Geometry: final body of the model. Coordinates: model frame, mm. Face numbers are marked on the shaded views. A direction names the side the tool comes from. Round coordinates to 2 decimals unless told otherwise and drop trailing zeros. Loops run counter-clockwise (first coordinate to the right, second up) from the corner with the lowest first, then second, coordinate; pieces in that order, holes last. Notation, with made-up numbers: (-31, 84.5) -> (1, 84.5) arc R11 ccw to (1, 100.5) -> close; hole circle Ø6 at (70.25, 56). An arc over 180 degrees is marked (long way). Answer in a Markdown table with one row per item.
```python
from build123d import *

# Parameters (mm, degrees)
SKETCH2_R           = 1.5
BOSS_EXTRUDE1_DEPTH = 10.5
SKETCH3_R           = 8
CUT_EXTRUDE1_DEPTH  = 4.5
SKETCH5_R           = 1.5
CUT_EXTRUDE3_DEPTH  = 22.113593143
CUT_EXTRUDE2_START  = -3
SKETCH4_R           = 8
CUT_EXTRUDE2_DEPTH  = 3


with BuildPart() as part:
    # Sketch2 → Boss-Extrude1 (new body)
    with BuildSketch(Plane.XY):
        with BuildLine():
            Line((7.937253933, 9), (14, 9))
            Line((14, 9), (14, -9))
            Line((14, -9), (7.937253933, -9))
            ThreePointArc((7.937253933, -9), (6.576406328, -10.037473776), (5.081826677, -10.870834265))
            Line((5.081826677, -10.870834265), (5.081826677, -16))
            Line((5.081826677, -16), (0, -16))
            Line((0, -16), (0, -9))
            Line((0, -9), (0, -6))
            ThreePointArc((0, -6), (6, 0), (0, 6))
            Line((0, 6), (0, 9))
            Line((0, 9), (0, 16))
            Line((0, 16), (5.081826677, 16))
            Line((5.081826677, 16), (5.081826677, 10.870834265))
            ThreePointArc((5.081826677, 10.870834265), (6.576406328, 10.037473776), (7.937253933, 9))
        make_face()
        with Locations(Location((10, 5, 0), (0, 0, 180))):
            Circle(SKETCH2_R, mode=Mode.SUBTRACT)
        with Locations(Location((10, -5, 0), (0, 0, 180))):
            Circle(SKETCH2_R, mode=Mode.SUBTRACT)
    extrude(amount=BOSS_EXTRUDE1_DEPTH)

    # Sketch3 → Cut-Extrude1 (cut)
    with BuildSketch(Plane.XY.offset(10.5)):
        Circle(SKETCH3_R)
    extrude(amount=-CUT_EXTRUDE1_DEPTH, mode=Mode.SUBTRACT)

    # Sketch5 → Cut-Extrude3 (cut, through all)
    with BuildSketch(Plane(origin=(5.081826677, 0, 0), x_dir=(0, 0, -1), z_dir=(1, 0, 0))):
        with Locations(Location((-5.25, 13, 0), (0, 0, 90))):
            Circle(SKETCH5_R)
        with Locations(Location((-5.25, -13, 0), (0, 0, 90))):
            Circle(SKETCH5_R)
    extrude(amount=-CUT_EXTRUDE3_DEPTH, mode=Mode.SUBTRACT)

    # Sketch4 → Cut-Extrude2 (cut)
    with BuildSketch(Plane(origin=(0, 0, 0), x_dir=(-1, 0, 0), z_dir=(0, 0, -1)).offset(CUT_EXTRUDE2_START)):
        Circle(SKETCH4_R)
    extrude(amount=CUT_EXTRUDE2_DEPTH, mode=Mode.SUBTRACT)


solid = part.part
```
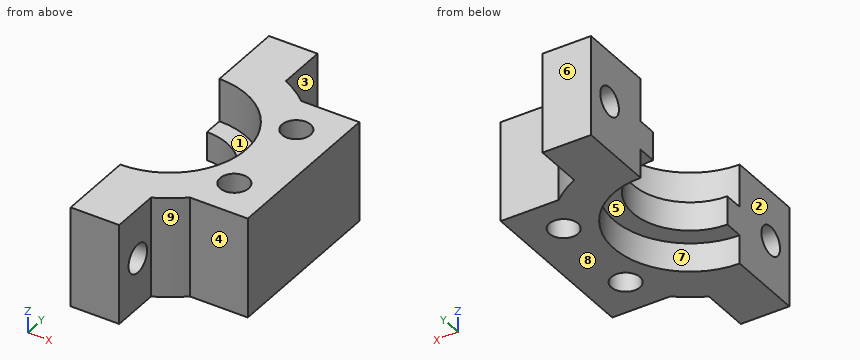
Item 1: Cut plane C-C (x = 10). Output: boundary loops of the cut face in (y, z), then the cut area to 3 significant figures.
Answer:
| item | result |
|---|---|
| outline | (-9, 0) -> (-6.5, 0) -> (-6.5, 10.5) -> (-9, 10.5) -> close; (-3.5, 0) -> (3.5, 0) -> (3.5, 10.5) -> (-3.5, 10.5) -> close; (6.5, 0) -> (9, 0) -> (9, 10.5) -> (6.5, 10.5) -> close |
| area | 126 mm² |
Item 2: Pin query (flat end, axial travel): pin 1 Ø4 at (y, z) = (-13.5, 3.5) entering from +X; pin 2 Ø3 at (x, z) = (10.5, 6.5) entering from +Y; pin 3 Ø5 at (y, z) = (-13, 5.25) entering from -X; pin 4 Ø6 at (y, z) = (-1.5, 3.5) entering from -X. Return the tip coordinate at first contact, or that it passes through.
Answer:
| item | result |
|---|---|
| pin 1 | stops at x = 5.08 |
| pin 2 | stops at y = 9 |
| pin 3 | stops at x = 0 |
| pin 4 | stops at x = 3.97 |
Item 3: Cut plane D-D (y = 13). Output: boundary loops of the cut face in (x, z), then the cut area to 3 significant figures.
Answer:
| item | result |
|---|---|
| outline | (0, 0) -> (5.08, 0) -> (5.08, 3.75) -> (0, 3.75) -> close; (0, 6.75) -> (5.08, 6.75) -> (5.08, 10.5) -> (0, 10.5) -> close |
| area | 38.1 mm² |
Item 4: Draft query along Y for the marked faces 6, 7, 8 and 9. Return one class per face: pulls with the +Y half, pulls with the -Y half, needs draft (parallel to the pull), parting line crosses it, or undercut.
Answer:
| item | result |
|---|---|
| face 6 | pulls with the +Y half |
| face 7 | undercut |
| face 8 | needs draft |
| face 9 | pulls with the -Y half |
Item 5: Reachability of the marked faces 1, 2, 3, 4 and 5 from +Z, -Z, +X, -X, +Y, -Y: full face, straight path, thin tool, end or side. Return the list, or none.
Answer:
| item | result |
|---|---|
| face 1 | +Z, -X |
| face 2 | +Z, -Z, -X, +Y, -Y |
| face 3 | +Z, -Z, +X, +Y |
| face 4 | +Z, -Z, +X, -Y |
| face 5 | -Z, -X |
Item 6: Cut plane A-A (z = 5.25). Output: boundary loops of the cut face in (x, y), then the cut area to 3 significant figures.
Answer:
| item | result |
|---|---|
| outline | (0, -16) -> (5.08, -16) -> (5.08, -14.5) -> (0, -14.5) -> close; (0, -11.5) -> (5.08, -11.5) -> (5.08, -10.87) arc R12 ccw to (7.94, -9) -> (14, -9) -> (14, 9) -> (7.94, 9) arc R12 ccw to (5.08, 10.87) -> (5.08, 11.5) -> (0, 11.5) -> (0, 6) arc R6 cw to (0, -6) -> close; (0, 14.5) -> (5.08, 14.5) -> (5.08, 16) -> (0, 16) -> close; hole circle Ø3 at (10, -5); hole circle Ø3 at (10, 5) |
| area | 228 mm² |
Item 7: Line query: probe 1 along Y at (x, z) = (10, 6.5); probe 2 along Z at (x, y) = (1.4, 13); probe 3 along Y at (x, z) = (5, 5.5). Output: solid intervals per line, ascending. Write a range as [from, to].
Answer:
| item | result |
|---|---|
| probe 1 | y = [-9, -6.5], [-3.5, 3.5], [6.5, 9] |
| probe 2 | z = [0, 3.75], [6.75, 10.5] |
| probe 3 | y = [-16, -14.48], [-11.52, -3.32], [3.32, 11.52], [14.48, 16] |
Item 8: Cut plane B-B (x = 2.5). Output: boundary loops of the cut face in (y, z).
Answer:
| item | result |
|---|---|
| outline | (-16, 0) -> (-7.6, 0) -> (-7.6, 3) -> (-5.45, 3) -> (-5.45, 6) -> (-7.6, 6) -> (-7.6, 10.5) -> (-16, 10.5) -> close; (5.45, 3) -> (7.6, 3) -> (7.6, 0) -> (16, 0) -> (16, 10.5) -> (7.6, 10.5) -> (7.6, 6) -> (5.45, 6) -> close; hole circle Ø3 at (-13, 5.25); hole circle Ø3 at (13, 5.25) |
